from build123d import *

# Parameters (mm, degrees)
PAD_DEPTH    = 15
SKETCH001_R  = 2
POCKET_DEPTH = 15
CHAMFER_SIZE = 1.5
FILLET_R     = 2


with BuildPart() as part:
    # Sketch → Pad (new body)
    with BuildSketch(Plane.XZ):
        with BuildLine():
            Line((0, 0), (30, 0))
            Line((30, 0), (30, 7))
            ThreePointArc((30, 7), (27.656854, 12.656854), (22, 15))
            Line((22, 15), (22, 13))
            Line((22, 13), (18.5, 13))
            Line((18.5, 13), (18.5, 15))
            Line((18.5, 15), (13.5, 15))
            Line((13.5, 15), (13.5, 13))
            Line((13.5, 13), (10, 13))
            Line((10, 13), (10, 15))
            Line((10, 15), (5, 15))
            Line((5, 15), (5, 13))
            Line((5, 13), (0, 13))
            Line((0, 13), (0, 0))
        make_face()
    extrude(amount=PAD_DEPTH)

    # Sketch001 (on Face1 of Pad) → Pocket (cut)
    with BuildSketch(Plane(origin=(0, 0, 0), x_dir=(1, 0, 0), z_dir=(0, 0, -1))):
        with Locations((7.5, 7.5)):
            Circle(SKETCH001_R)
        with Locations((20.5, 7.5)):
            Circle(SKETCH001_R)
    extrude(amount=-POCKET_DEPTH, mode=Mode.SUBTRACT)

    # Chamfer
    chamfer_edges = [part.edges().sort_by_distance(p)[0] for p in [
        (5.5, -7.5, 0),
        (18.5, -7.5, 0),
    ]]
    chamfer(chamfer_edges, length=CHAMFER_SIZE)

    # Fillet
    fillet_edges = [part.edges().sort_by_distance(p)[0] for p in [
        (0, -15, 6.5),
        (0, 0, 6.5),
        (0, -7.5, 0),
        (15, -15, 0),
        (15, 0, 0),
    ]]
    fillet(fillet_edges, radius=FILLET_R)


solid = part.part
Here's how the part is built. I have some questions about the finished solid (model axes, mm). A direction names the side the tool comes from. Give positions to 0.01 mm unless a question says otherwise; leave off trailing zeros. Loops run counter-clockwise (first coordinate to the right, second up) from the corner with the lowest first, then second, coordinate; pieces in that order, holes last. Notation, with made-up numbers: (70, 8.25) -> (115, 8.25) arc R20 cw to (115, 34.25) -> close; hole circle Ø4 at (-18.5, -20). An arc over 180 degrees is marked (long way). One line per item, written item: value.
Q1. Suppose I cut it at D-D on x = 20.5. Please give me the cut outline in (y, z), then the cut area to 3 significant figures.
Answers follow:
outline: (-15, 2) arc R2 ccw to (-13, 0) -> (-11, 0) -> (-9.5, 1.5) -> (-9.5, 13) -> (-15, 13) -> close; (-5.5, 1.5) -> (-4, 0) -> (-2, 0) arc R2 ccw to (0, 2) -> (0, 13) -> (-5.5, 13) -> close
area: 139 mm^2
Q2. Suppose I cut it at B-B on z = 6. Please give me the cut outline in (x, y), then the cut area to 3 significant figures.
Answers follow:
outline: (0, -13) arc R2 ccw to (2, -15) -> (30, -15) -> (30, 0) -> (2, 0) arc R2 ccw to (0, -2) -> close; hole circle Ø4 at (7.5, -7.5); hole circle Ø4 at (20.5, -7.5)
area: 423 mm^2
Q3. I'm going to push flat-ended pins straight in: pin 1 Ø6 at (y, z) = (-6, 11) entering from +X; pin 2 Ø2 at (x, y) = (10, -9) entering from -Z; pin 3 Ø0.6 at (y, z) = (-4, 14) entering from -X; pin 4 Ø2.5 at (x, y) = (3.5, -7.5) entering from +Z. Where does each tip first touch, or does it pass through?
Answers follow:
pin 1: x = 29.94
pin 2: z = 0
pin 3: x = 5
pin 4: z = 13
Q4. We'd pull the mould along X, two halves only. Please class faces 1 (the face through (5, -7, 14)), 2 (the face through (16, 0, 9)), 3 (the face through (22.408, -8.101, 8.156)): pulls with the +X half, pulls with the -X half, needs draft (parallel to the pull), parting line crosses it, or undercut.
Answers follow:
face 1: pulls with the -X half
face 2: needs draft
face 3: undercut
Q5. Suppose I cut it at C-C on y = -2.75. Please give me the cut outline in (x, z).
Answers follow:
outline: (0, 2) arc R2 ccw to (2, 0) -> (30, 0) -> (30, 7) arc R8 ccw to (22, 15) -> (22, 13) -> (18.5, 13) -> (18.5, 15) -> (13.5, 15) -> (13.5, 13) -> (10, 13) -> (10, 15) -> (5, 15) -> (5, 13) -> (0, 13) -> close
Q6. Suppose I cut it at A-A on x = 7.5. Please give me the cut outline in (y, z), then the cut area to 3 significant figures.
Answers follow:
outline: (-15, 2) arc R2 ccw to (-13, 0) -> (-11, 0) -> (-9.5, 1.5) -> (-9.5, 15) -> (-15, 15) -> close; (-5.5, 1.5) -> (-4, 0) -> (-2, 0) arc R2 ccw to (0, 2) -> (0, 15) -> (-5.5, 15) -> close
area: 161 mm^2
Q7. If I drill on line 1 along Y through (x, z) = (20.5, 5.5); line 2 along X through (y, z) = (-7.5, 6.5); line 3 along X through (y, z) = (-6.25, 13.5), over which ranges is the centre line in solid material (lowest first)?
Answers follow:
line 1: -15 to -9.5, -5.5 to 0
line 2: 0 to 5.5, 9.5 to 18.5, 22.5 to 30
line 3: 5 to 5.94, 9.06 to 10, 13.5 to 18.5, 22.06 to 26.66
Q8. On a 3-axis mill with a long thin cutter (end or side, diameter ignored), from which of +Z, -Z, +X, -X, +Y, -Y can I reach the whole of each face in a straight line? I mean faces 4 (the face through (16.2, -14.4, 0.57)), 5 (the face through (22, -12, 14)). Say none if no direction works.
Answers follow:
face 4: -Z, +X, -X, -Y
face 5: +Z, +Y, -Y
